Check sheet for the modelled part. Datum: model origin and axes. Units: mm. A direction names the side the tool comes from. Round coordinates to 2 decimals unless told otherwise and drop trailing zeros. Write each loop counter-clockwise with the first axis right and the second up, starting at its lowest first coordinate (ties: lowest second). Pieces come first, ordered by that corner, then holes. Notation, with made-up numbers: (12, 44.5) -> (60, 44.5) arc R14 ccw to (60, 51.5) -> close; hole circle Ø10 at (-30.5, 75.5). An arc over 180 degrees is marked (long way). One line per item, written item: value. Start each with the question number.
```python
from build123d import *

# Parameters (mm, degrees)
SKETCH1_W                 = 18.25
SKETCH1_H                 = 25
BOSS_EXTRUDE1_DEPTH       = 8
M10X1_0_TAPPED_HOLE1_D    = 9
SKETCH7_R                 = 3.375
SKETCH7_R_2               = 0.9906
CUT_EXTRUDE2_DEPTH        = 19.25
M3X0_5_TAPPED_HOLE1_D     = 2.5
M3X0_5_TAPPED_HOLE1_DEPTH = 6.35
M3X0_5_TAPPED_HOLE1_TIP   = 0.751075774


with BuildPart() as part:
    # Sketch1 → Boss-Extrude1 (new body)
    with BuildSketch(Plane(origin=(0, 0, 0), x_dir=(1, 0, 0), z_dir=(0, 1, 0))):
        with Locations((0, -5.5)):
            Rectangle(SKETCH1_W, SKETCH1_H)
    extrude(amount=BOSS_EXTRUDE1_DEPTH)

    # M10x1.0 Tapped Hole1 (through all)
    with Locations(Plane(origin=(0, 8, 0), x_dir=(-1, 0, 0), z_dir=(0, 1, 0))):
        with Locations((0, 0)):
            Hole(M10X1_0_TAPPED_HOLE1_D / 2)

    # Sketch7 → Cut-Extrude2 (cut, through all)
    with BuildSketch(Plane(origin=(9.125, 0, 0), x_dir=(0, 0, -1), z_dir=(1, 0, 0))):
        with Locations((-13.336186812, 4)):
            Circle(SKETCH7_R)
        with Locations((-7.3575, 4)):
            Circle(SKETCH7_R_2)
    extrude(amount=-CUT_EXTRUDE2_DEPTH, mode=Mode.SUBTRACT)

    # M3x0.5 Tapped Hole1
    with Locations(Plane(origin=(9.125, 0, 0), x_dir=(0, 0, -1), z_dir=(1, 0, 0))):
        with Locations((0, 4)):
            Hole(M3X0_5_TAPPED_HOLE1_D / 2, depth=M3X0_5_TAPPED_HOLE1_DEPTH)
            with Locations((0, 0, -(M3X0_5_TAPPED_HOLE1_DEPTH + M3X0_5_TAPPED_HOLE1_TIP / 2))):  # 118° drill point
                Cone(0, M3X0_5_TAPPED_HOLE1_D / 2, M3X0_5_TAPPED_HOLE1_TIP, mode=Mode.SUBTRACT)


solid = part.part
```
1. Access from +Z, -Z, +X, -X, +Y, -Y to the whole of each face (thin tool, end or side, straight path). Record for faces 5 (the face through (0, 4, -7)), 6 (the face through (6.69, 2.78, -0.27)).
2. Cross-section at B-B (y = 1). Record the cut outline in (x, z) (3 decimals), plus the area to 3 significant figures.
3. Cross-section at C-C (z = 0). Record the cut outline in (x, y) (3 decimals), plus the area to 3 significant figures.
4. Release check for a two-part mould opening along X. For faces 1 (the face through (-0.59, 3.94, 4.46)), 2 (the face through (9.125, 4, 6)), 3 (the face through (-9.125, 4, 6)), 4 (the face through (0, 0, 5)) record: +X half, -X half, draft (parallel to the pull), parting line (faces both ways), or undercut.
5. Cross-section at D-D (y = 4). Record the cut outline in (x, z) (3 decimals), plus the area to 3 significant figures.
6. Material ranges on probe 1 along Z at (x, y) = (0.5, 7); probe 2 along Z at (x, y) = (6.5, 6); probe 3 along Y at (x, z) = (7, 0.5), recorded low to high.
7. Cross-section at A-A (x = 0). Give the number of separate pieces and of enclosed holes in the cut face, plus the area to 3 significant figures.
Working result:
1. face 5: -Z, +X, -X, +Y, -Y
1. face 6: +X
2. outline: (-9.125, -7) -> (9.125, -7) -> (9.125, 11.79) -> (-9.125, 11.79) -> close; (-9.125, 14.882) -> (9.125, 14.882) -> (9.125, 18) -> (-9.125, 18) -> close; hole circle Ø9 at (0, 0)
2. area: 336 mm^2
3. outline: (-9.125, 0) -> (-4.5, 0) -> (-4.5, 8) -> (-9.125, 8) -> close; (4.5, 0) -> (9.125, 0) -> (9.125, 2.75) -> (4.5, 2.75) -> close; (4.5, 5.25) -> (9.125, 5.25) -> (9.125, 8) -> (4.5, 8) -> close
3. area: 62.4 mm^2
4. face 1: undercut
4. face 2: +X half
4. face 3: -X half
4. face 4: draft
5. outline: (-9.125, -7) -> (9.125, -7) -> (9.125, -1.25) -> (4.323, -1.25) arc R4.5 cw (long way) to (4.323, 1.25) -> (9.125, 1.25) -> (9.125, 6.367) -> (-9.125, 6.367) -> close; (-9.125, 8.348) -> (9.125, 8.348) -> (9.125, 9.961) -> (-9.125, 9.961) -> close; (-9.125, 16.711) -> (9.125, 16.711) -> (9.125, 18) -> (-9.125, 18) -> close
5. area: 222 mm^2
6. probe 1: z = -7 to -4.47, 4.47 to 11.79, 14.88 to 18
6. probe 2: z = -7 to 10.62, 16.05 to 18
6. probe 3: y = 0 to 2.85, 5.15 to 8
7. separate pieces: 2
7. enclosed holes: 2
7. area: 89.1 mm^2
